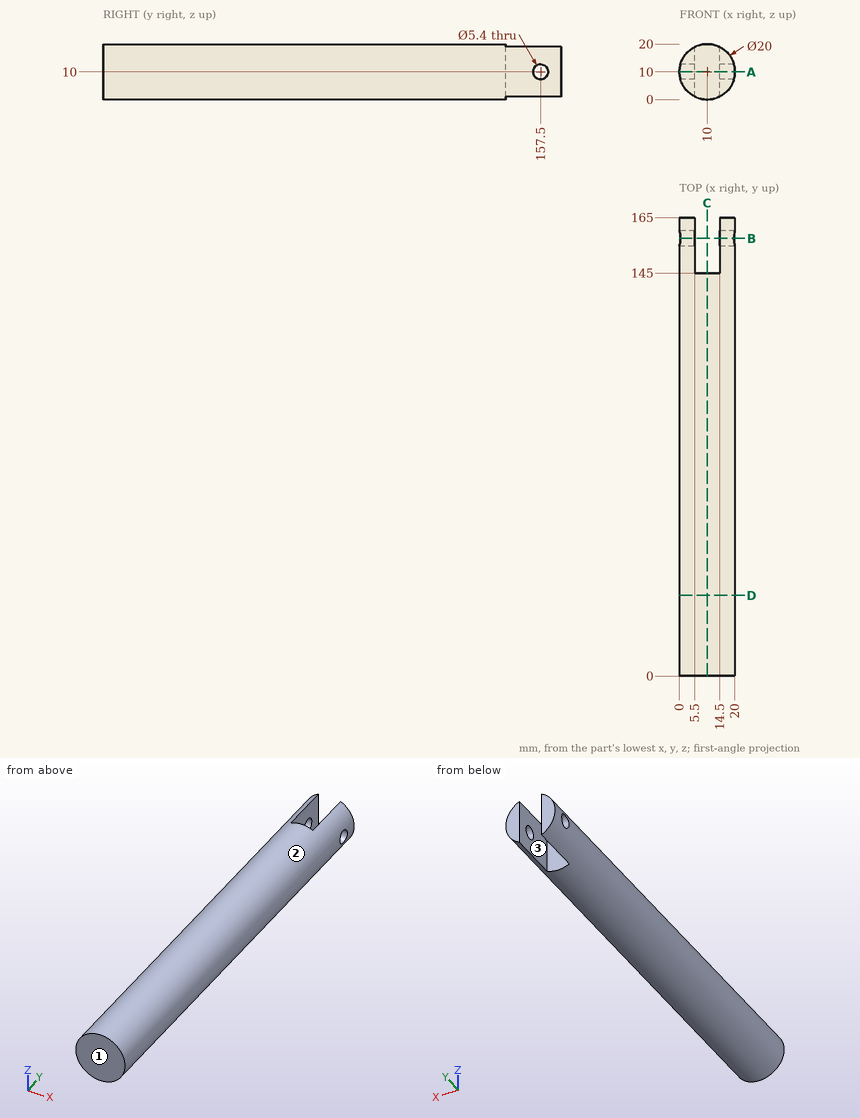
Verification items for this drawing (mm, ordinates from the low corner). Coordinates: 2 decimals unless noted, no trailing zeros. Order: outer loops, then holes, each group sorted by start corner. A loop starts at its lowest first (then second) coordinate and runs counter-clockwise, first axis right, second up. Notation, with made-up numbers: (21.25, 60.5) -> (58.25, 60.5) arc R34 cw to (58.25, 99.5) -> close; hole circle Ø2 at (81, 53.5). An arc over 180 degrees is marked (long way). Answer as CSV lines item,"result". Start each with the question number.
1) Cross-section at C-C, the plane x = 10. Record the boundary of the cut face in (y, z).
2) Cross-section at A-A, the plane z = 10. Record the boundary of the cut face in (x, y).
3) Cross-section at D-D, the plane y = 29. Record the boundary of the cut face in (x, z), then the cut area to 3 significant figures.
4) Material ranges on L1, parallel to X at y = 56.5, z = 10.25; L2, parallel to Z at x = 1.65, y = 157.5; L3, parallel to Y at x = 13, z = 17, recorded low to high. Write a range as [from, to].
5) Release check for a two-part mould opening along X. For the marked faces 1, 2 and 3 record: released by +X, released by -X, zero draft, split by the parting line, or undercut.
6) Cross-section at B-B, the plane y = 157.5. Record the boundary of the cut face in (x, z), then the cut area to 3 significant figures.
7) Gauge pin test, flat ends, axial feed: pin 1 Ø6 at (y, z) = (67, 17.5) entering from -X; pin 2 Ø3 at (x, y) = (3, 78) entering from -Z; pin 3 Ø1 at (x, y) = (14.5, 47.5) entering from -Z; pin 4 Ø6 at (y, z) = (157.5, 10) entering from +X. Record the tip position at first contact, or that the pin passes through.
Conclusion:
1,outline,"(0, 0) -> (145, 0) -> (145, 20) -> (0, 20) -> close"
2,outline,"(0, 0) -> (20, 0) -> (20, 154.8) -> (14.5, 154.8) -> (14.5, 145) -> (5.5, 145) -> (5.5, 154.8) -> (0, 154.8) -> close; (0, 160.2) -> (5.5, 160.2) -> (5.5, 165) -> (0, 165) -> close; (14.5, 160.2) -> (20, 160.2) -> (20, 165) -> (14.5, 165) -> close"
3,outline,"circle Ø20 at (10, 10)"
3,area,"314 mm²"
4,L1,"x = [0, 20]"
4,L2,"z = [4.5, 7.3], [12.7, 15.5]"
4,L3,"y = [0, 145]"
5,face 1,"zero draft"
5,face 2,"split by the parting line"
5,face 3,"undercut"
6,outline,"(0.37, 7.3) arc R10 ccw to (5.5, 1.07) -> (5.5, 7.3) -> close; (0.37, 12.7) -> (5.5, 12.7) -> (5.5, 18.93) arc R10 ccw to start; (14.5, 1.07) arc R10 ccw to (19.63, 7.3) -> (14.5, 7.3) -> close; (14.5, 12.7) -> (19.63, 12.7) arc R10 ccw to (14.5, 18.93) -> close"
6,area,"82.4 mm²"
7,pin 1,"stops at x = 1.07"
7,pin 2,"stops at z = 1.65"
7,pin 3,"stops at z = 0.83"
7,pin 4,"stops at x = 20"
